from build123d import *

# Parameters (mm, degrees)
ESQUISSE1_R        = 10.5
ESQUISSE1_R_2      = 0.8
ESQUISSE1_R_3      = 1.5
BOSS_EXTRU_1_DEPTH = 3
ESQUISSE3_R        = 2
ESQUISSE3_R_2      = 1.5
BOSS_EXTRU_2_DEPTH = 3.7
CONG_1_R           = 1


with BuildPart() as part:
    # Esquisse1 → Boss.-Extru.1 (new body)
    with BuildSketch(Plane.XY):
        with Locations((-15.570186162, 4.534749907)):
            Circle(ESQUISSE1_R)
        with Locations((-12.070186162, 12.834749907)):
            Circle(ESQUISSE1_R_2, mode=Mode.SUBTRACT)
        with Locations((-15.570186162, 4.534749907)):
            Circle(ESQUISSE1_R_3, mode=Mode.SUBTRACT)
        with Locations((-7.270186162, 4.534749907)):
            Circle(ESQUISSE1_R_2, mode=Mode.SUBTRACT)
        with Locations((-15.570186162, 12.834749907)):
            Circle(ESQUISSE1_R_2, mode=Mode.SUBTRACT)
        with Locations((-23.870186162, 4.534749907)):
            Circle(ESQUISSE1_R_2, mode=Mode.SUBTRACT)
        with Locations((-15.570186162, -3.765250093)):
            Circle(ESQUISSE1_R_2, mode=Mode.SUBTRACT)
        with Locations((-19.070186162, 12.834749907)):
            Circle(ESQUISSE1_R_2, mode=Mode.SUBTRACT)
        with Locations((-19.070186162, -3.765250093)):
            Circle(ESQUISSE1_R_2, mode=Mode.SUBTRACT)
        with Locations((-12.070186162, -3.765250093)):
            Circle(ESQUISSE1_R_2, mode=Mode.SUBTRACT)
        with Locations((-7.270186162, 8.034749907)):
            Circle(ESQUISSE1_R_2, mode=Mode.SUBTRACT)
        with Locations((-7.270186162, 1.034749907)):
            Circle(ESQUISSE1_R_2, mode=Mode.SUBTRACT)
        with Locations((-23.870186162, 1.034749907)):
            Circle(ESQUISSE1_R_2, mode=Mode.SUBTRACT)
        with Locations((-23.870186162, 8.034749907)):
            Circle(ESQUISSE1_R_2, mode=Mode.SUBTRACT)
    extrude(amount=BOSS_EXTRU_1_DEPTH)

    # Esquisse3 → Boss.-Extru.2 (add)
    with BuildSketch(Plane.XY.offset(3)):
        with Locations((-15.570186162, 4.534749907)):
            Circle(ESQUISSE3_R)
        with Locations((-15.570186162, 4.534749907)):
            Circle(ESQUISSE3_R_2, mode=Mode.SUBTRACT)
    extrude(amount=BOSS_EXTRU_2_DEPTH)

    # Congé1
    cong_1_edges = [part.edges().sort_by_distance(p)[0] for p in [
        (-17.570186162, 4.534749907, 3),
    ]]
    fillet(cong_1_edges, radius=CONG_1_R)


solid = part.part
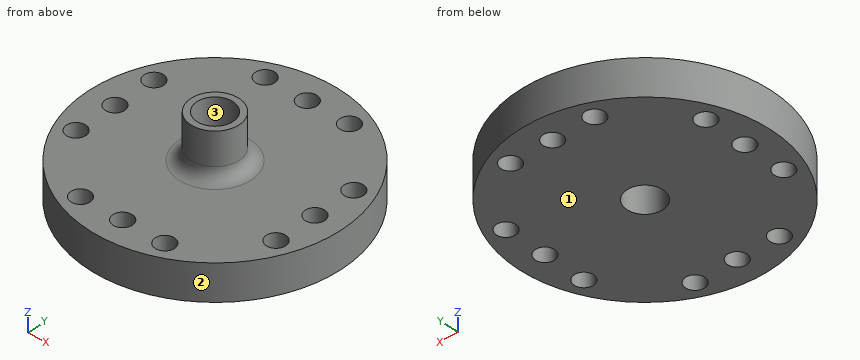
Geometry: final body of the model. Coordinates: model frame, mm. Face numbers are marked on the shaded views. Round coordinates to 2 decimals unless told otherwise and drop trailing zeros. Loops run counter-clockwise (first coordinate to the right, second up) from the corner with the lowest first, then second, coordinate; pieces in that order, holes last.
Q1. Section B-B on x = -19. Return loops of the section in (y, z), plus the area to 3 significant figures.
Q2. Section A-A on z = 1.25. State how many separate pieces and enclosed holes the cut face has, plus the area to 3 significant figures.
Q3. Pull-direction query (Y, two-part tool) for the marked faces 1, 2 and 3; classes: released by +Y, released by -Y, zero draft, split by the parting line, or undercut.
Q4. Section D-D on z = 6. Return loops of the section in (x, y), plus the area to 3 significant figures.
Q5. Material intervals for L1, parallel to X at y = 4.5, z = 2; L2, parallel to Y at x = -11.75, z = 2.5; L3, parallel to X at y = 12.5, z = 0.75, sorted ascending.
Q6. Pin query (flat end, axial travel): P1, Ø3, axis at y = -1.5, z = 3, coming from the -X side; P2, Ø2.5, axis at x = -12.07, y = 12.83, coming from the +Z side; P3, Ø1, axis at x = -8.5, z = 1.5, coming from the -Y side. Return the tip coordinate at first contact, or that it passes through.
Evaluation:
1. outline: (-5.39, 0) - (-4.56, 0) - (-4.56, 3) - (-5.39, 3) - close; (-2.97, 0) - (12.04, 0) - (12.04, 3) - (-2.97, 3) - close; (13.63, 0) - (14.46, 0) - (14.46, 3) - (13.63, 3) - close
1. area: 50.0 mm2
2. separate pieces: 1
2. enclosed holes: 13
2. area: 315 mm2
3. face 1: zero draft
3. face 2: split by the parting line
3. face 3: undercut
4. outline: circle Ø4 at (-15.57, 4.53); hole circle Ø3 at (-15.57, 4.53)
4. area: 5.50 mm2
5. L1: x = -26.07 to -24.67, -23.07 to -17.07, -14.07 to -8.07, -6.47 to -5.07
5. L2: y = -5.25 to -4.5, -3.03 to 12.1, 13.57 to 14.32
5. L3: x = -22.41 to -19.8, -18.34 to -16.3, -14.84 to -12.8, -11.34 to -8.73
6. P1: stops at x = -25.04
6. P2: stops at z = 3
6. P3: stops at y = -3.66
